from build123d import *

# Parameters (mm, degrees)
F0_R             = 15
F1_DEPTH         = 25.4
F2_SIZE          = 3
F3_SIZE          = 2
F4_R             = 5
F5_DEPTH         = 2.5
F6_R             = 3
F7_DEPTH         = 25
F10_DEPTH        = 7.53734
F10_COPIES_COUNT = 9


# Not quite as in the source:
# - a pattern or mirror of a feature is missing from the dataset's text; its kind, count and spacing are read off the source's solid


with BuildPart() as f1:
    # F0 (on Top) → F1 (new body)
    with BuildSketch(Plane.XY):
        Circle(F0_R)
    extrude(amount=F1_DEPTH)

    # F2
    f2_edges = [f1.edges().sort_by_distance(p)[0] for p in [
        (-15, 0, 25.4),
    ]]
    chamfer(f2_edges, length=F2_SIZE)

    # F3
    f3_edges = [f1.edges().sort_by_distance(p)[0] for p in [
        (-15, 0, 0),
    ]]
    chamfer(f3_edges, length=F3_SIZE)

    # F4 (on face) → F5 (cut)
    with BuildSketch(Plane.XY.offset(25.4)):
        Circle(F4_R)
    extrude(amount=-F5_DEPTH, mode=Mode.SUBTRACT)

    # F6 (on face) → F7 (join)
    with BuildSketch(Plane.XY.offset(22.9)):
        Circle(F6_R)
    extrude(amount=F7_DEPTH)

    # F9 (on offset) → F10 (cut)
    with BuildSketch(Plane.XZ.offset(15)):
        with BuildLine():
            Line((1.0176621057, 25.4637251124), (-0.9823378943, 25.4637251124))
            Line((-0.9823378943, 25.4637251124), (-0.9823378943, 21.4637251124))
            ThreePointArc((-0.9823378943, 21.4637251124), (0.0176621057, 21.1957759199), (1.0176621057, 21.4637251124))
            Line((1.0176621057, 21.4637251124), (1.0176621057, 25.4637251124))
        make_face()
    f10 = extrude(amount=-F10_DEPTH, mode=Mode.SUBTRACT)

    # F10_copies: F10 ×9 about axis
    f10_copies_axis = Axis((0, 0, 0), (0, 0, 1))
    for i in range(1, F10_COPIES_COUNT):
        add(f10.rotate(f10_copies_axis, i * 360 / F10_COPIES_COUNT), mode=Mode.SUBTRACT)


solid = f1.part
Geometry: final body of the model. Coordinates: model frame, mm. A direction names the side the tool comes from. Give positions to 0.01 mm unless a question says otherwise; leave off trailing zeros. Order: outer loops, then holes, each group sorted by start corner. A loop starts at its lowest first (then second) coordinate and runs counter-clockwise, first axis right, second up. Notation, with made-up numbers: (52, -10) -> (71, -10) arc R28 ccw to (71, 12) -> close; hole circle Ø9 at (56.25, -21). An arc over 180 degrees is marked (long way). Write each question's results on one line, items separated by ' | '.
1) Draft query along Y for faces 3 (the face through (3.857, 10.605, 21.196)), 4 (the face through (0, 0, 47.9)), 5 (the face through (0, 13.5, 23.9)). Return one class per face: released by +Y, released by -Y, zero draft, split by the parting line, or undercut.
Geometry says:
face 3: undercut | face 4: zero draft | face 5: released by +Y
2) Line query: line 1 along Y through (x, z) = (0, 23); line 2 along Y through (x, z) = (0, 24.2); line 3 along Z through (x, y) = (3.5, 2). Output: solid intervals per line, ascending.
Geometry says:
line 1: y = -7.46 to -5, -3 to 3, 5 to 14.4 | line 2: y = -7.46 to -5, -3 to 3, 5 to 13.2 | line 3: z = 0 to 22.9
3) Cut plane C-C (x = 0). Output: boundary loops of the cut face in (y, z), and give its area (3 significant figures).
Geometry says:
outline: (-15, 2) -> (-13, 0) -> (13, 0) -> (15, 2) -> (15, 22.4) -> (12, 25.4) -> (5, 25.4) -> (5, 22.9) -> (3, 22.9) -> (3, 47.9) -> (-3, 47.9) -> (-3, 22.9) -> (-5, 22.9) -> (-5, 25.4) -> (-7.46, 25.4) -> (-7.46, 21.2) -> (-15, 21.2) -> close | area: 847 mm²
4) First-contact query: pin 1 Ø6 at (x, z) = (8, 21.5) entering from +Y; pin 2 Ø6 at (x, y) = (3.5, 7) entering from +Z; pin 3 Ø12 at (x, z) = (5, 35.5) entering from -Y. Flat tips, straight axial feed; report the tip coordinate or a pass-through.
Geometry says:
pin 1: stops at y = 14.14 | pin 2: stops at z = 25.4 | pin 3: stops at y = -3
5) Cut plane B-B (z = 23.5). Give the number of separate pieces and of enclosed holes in the cut face, and give its area (3 significant figures).
Geometry says:
separate pieces: 2 | enclosed holes: 1 | area: 441 mm²
6) Cut plane A-A (z = 8). Output: boundary loops of the cut face in (x, y), and give its area (3 significant figures).
Geometry says:
outline: circle Ø30 at (0, 0) | area: 707 mm²
7) Set-up query: faces 1 (the face through (-9.544, 4.335, 23.404)), 2 (the face through (-8.64, 10.35, 23.92)). Return all of +Z, -Z, +X, -X, +Y, -Y with unobstructed straight access to the full face (end or side cutting, diameter ignored); none if empty.
Geometry says:
face 1: +Z | face 2: +Z, -X, +Y
8) Cut plane D-D (z = 32). Output: boundary loops of the cut face in (x, y).
Geometry says:
outline: circle Ø6 at (0, 0)
